```python
from build123d import *

# Parameters (mm, degrees)
F0_W          = 28.3464
F0_H          = 2.54
F0_W_2        = 2.54
F1_DEPTH      = 43.18
F2_W          = 28.3464
F2_H          = 10.16
F3_DEPTH      = 2.54
F2_W_2        = 2.54
F2_H_2        = 2.54
F4_DEPTH      = 12.7
F5_DEPTH      = 25.4
F6_W          = 33.4264
F6_H          = 22.86
F7_DEPTH      = 12.7
F9_W          = 35.56
F9_H          = 27.94
F10_DEPTH     = 25.4
F11_W         = 35.56
F11_H         = 22.86
F12_DEPTH     = 12.7
F14_W         = 36.8241928518
F14_H         = 28.1280204654
F15_DEPTH     = 25.4
F17_DEPTH     = 12.7
F19_W         = 36.3356121816
F19_H         = 38.6965835933
F20_DEPTH     = 25.4
F21_T4_DEPTH  = 37.4897748093
F21_T10_DEPTH = 37.4897748093
F22_T4_DEPTH  = 41.4622128931
F22_T9_DEPTH  = 41.4622128931
F22_T15_DEPTH = 39.215050137
F22_T21_DEPTH = 39.215050137
F22_T26_DEPTH = 13.1188216118
F23_T4_DEPTH  = 41.4622128931
F23_T9_DEPTH  = 41.4622128931
F23_T14_DEPTH = 39.215050137
F24_W         = 28.3464
F24_H         = 2.54
F25_DEPTH     = 25.4


# Not quite as in the source:
# - a fillet or chamfer that OpenCascade refuses, or shapes differently, is made with other operations: its cross-section is extruded or revolved along the edge and cut away or added


with BuildPart() as f1:
    # F0 (on Front) → F1 (new body)
    with BuildSketch(Plane.XZ):
        with Locations((16.7132, 1.27)):
            Rectangle(F0_W, F0_H)
        with Locations((1.27, 1.27)):
            Rectangle(F0_W_2, F0_H)
        with Locations((32.1564, 1.27)):
            Rectangle(F0_W_2, F0_H)
    extrude(amount=F1_DEPTH)

    # F2 (on face) → F3 (cut)
    with BuildSketch(Plane.XY.offset(2.54)):
        Polygon((30.8864, 0), (2.54, 0), (2.54, -7.62), (2.54, -27.94), (30.8864, -27.94), (30.8864, -7.62), align=None)
        with Locations((16.7132, -35.56)):
            Rectangle(F2_W, F2_H)
    extrude(amount=-F3_DEPTH, mode=Mode.SUBTRACT)

    # F2 (on face) → F4 (join)
    with BuildSketch(Plane.XY.offset(2.54)):
        with Locations((1.27, -41.91)):
            Rectangle(F2_W_2, F2_H_2)
        with Locations((32.1564, -41.91)):
            Rectangle(F2_W_2, F2_H_2)
    extrude(amount=F4_DEPTH)

    # F2 (on face) → F5 (join)
    with BuildSketch(Plane.XY.offset(2.54)):
        Polygon((2.54, -7.62), (0, -7.62), (0, -40.64), (2.54, -40.64), (2.54, -30.48), (2.54, -27.94), align=None)
        Polygon((33.4264, -7.62), (30.8864, -7.62), (30.8864, -27.94), (30.8864, -30.48), (30.8864, -40.64), (33.4264, -40.64), align=None)
        with Locations((16.7132, -41.91)):
            Rectangle(F2_W, F2_H_2)
        with Locations((1.27, -41.91)):
            Rectangle(F2_W_2, F2_H_2)
        with Locations((32.1564, -41.91)):
            Rectangle(F2_W_2, F2_H_2)
    extrude(amount=-F5_DEPTH)

    # F6 (on face) → F7 (join)
    with BuildSketch(Plane.XZ.offset(43.18)):
        with Locations((16.7132, -11.43)):
            Rectangle(F6_W, F6_H)
    extrude(amount=F7_DEPTH)

    # F9 (on 3pt) → F10 (cut)
    with BuildSketch(Plane(origin=(0, -32.9960377358, 18.3311320755), x_dir=(-1, 0, 0), z_dir=(0, 0.8741572761, -0.4856429312))):
        with Locations((-17.78, -36.665337096)):
            Rectangle(F9_W, F9_H)
    extrude(amount=-F10_DEPTH, mode=Mode.SUBTRACT)

    # F11 (on face) → F12 (join)
    with BuildSketch(Plane.YZ.offset(33.4264)):
        with Locations((-25.4, -11.43)):
            Rectangle(F11_W, F11_H)
    extrude(amount=F12_DEPTH)

    # F14 (on 3pt) → F15 (cut)
    with BuildSketch(Plane(origin=(25.5428150943, 0, 14.1904528302), x_dir=(0, -1, 0), z_dir=(-0.8741572761, 0, -0.4856429312))):
        with Locations((24.8448457569, -30.2426330745)):
            Rectangle(F14_W, F14_H)
    extrude(amount=-F15_DEPTH, mode=Mode.SUBTRACT)

    # F16 (on face) → F17 (join)
    with BuildSketch(Plane(origin=(0, 0, 0), x_dir=(0, -1, 0), z_dir=(-1, 0, 0))):
        Polygon((40.64, -22.86), (40.64, 2.54), (7.62, 2.54), (7.62, 0), (7.62, -22.86), align=None)
    extrude(amount=F17_DEPTH)

    # F19 (on 3pt) → F20 (cut)
    with BuildSketch(Plane(origin=(-1.016, 0, 0.508), x_dir=(0, -1, 0), z_dir=(-0.894427191, 0, 0.4472135955))):
        with Locations((25.5430552643, -17.0687864302)):
            Rectangle(F19_W, F19_H)
    extrude(amount=F20_DEPTH, mode=Mode.SUBTRACT)

    # F21: chamfer of 5.08 on 2 edges, made by hand


with BuildPart() as f21_tool2:
    # F21_s3 → F21_t4 (new body)
    with BuildSketch(Plane(origin=(0, -29.228474159, -52.6112534862), x_dir=(1, 0, 0), z_dir=(0, 0.4856429312, 0.8741572761))):
        with BuildLine():
            Line((-0.1436840979, -32.522427085), (5.2236840979, -37.8897952809))
            Line((5.2236840979, -37.8897952809), (5.2236840979, -37.9913952809))
            ThreePointArc((5.2236840979, -37.9913952809), (2.611842049, -37.8477111829), (0, -37.8477111829))
            Line((0, -37.8477111829), (-0.1016, -37.7461111829))
            ThreePointArc((-0.1016, -37.7461111829), (-0.1016, -35.134269134), (-0.2452840979, -32.522427085))
            Line((-0.2452840979, -32.522427085), (-0.1436840979, -32.522427085))
        make_face()
    extrude(amount=F21_T4_DEPTH)

    split(bisect_by=Plane.XY.offset(-22.86), keep=Keep.TOP)

    split(bisect_by=Plane.XZ.offset(40.64), keep=Keep.TOP)


with BuildPart() as f1_1:
    add(f1.part)

    # F21_t1: cut F21_tool2
    add(f21_tool2.part, mode=Mode.SUBTRACT)


with BuildPart() as f21_tool8:
    # F21_s9 → F21_t10 (new body)
    with BuildSketch(Plane(origin=(0, -11.0218300314, -19.8392940565), x_dir=(1, 0, 0), z_dir=(0, -0.4856429312, -0.8741572761))):
        with BuildLine():
            Line((33.5700840979, 32.522427085), (28.2027159021, 37.8897952809))
            Line((28.2027159021, 37.8897952809), (28.2027159021, 37.9913952809))
            ThreePointArc((28.2027159021, 37.9913952809), (30.814557951, 37.8477111829), (33.4264, 37.8477111829))
            Line((33.4264, 37.8477111829), (33.528, 37.7461111829))
            ThreePointArc((33.528, 37.7461111829), (33.528, 35.134269134), (33.6716840979, 32.522427085))
            Line((33.6716840979, 32.522427085), (33.5700840979, 32.522427085))
        make_face()
    extrude(amount=F21_T10_DEPTH)

    split(bisect_by=Plane.XZ.offset(43.18), keep=Keep.TOP)

    split(bisect_by=Plane.XY.offset(-22.86), keep=Keep.TOP)


with BuildPart() as f1_2:
    add(f1_1.part)

    # F21_t7: cut F21_tool8
    add(f21_tool8.part, mode=Mode.SUBTRACT)

    # F22: chamfer of 5.08 on 2 edges, made by hand


with BuildPart() as f22_tool2:
    # F22_s3 → F22_t4 (new body)
    with BuildSketch(Plane(origin=(-17.5264653053, 0, -35.0529306106), x_dir=(0, 1, 0), z_dir=(0.4472135955, 0, 0.894427191))):
        Polygon((-40.64, -3.9440774674), (-35.56, 1.1359225326), (-40.64, 1.1359225326), align=None)
    extrude(amount=F22_T4_DEPTH)

    split(bisect_by=Plane.YZ, keep=Keep.BOTTOM)


with BuildPart() as f1_3:
    add(f1_2.part)

    # F22_t1: cut F22_tool2
    add(f22_tool2.part, mode=Mode.SUBTRACT)


with BuildPart() as f22_tool7:
    # F22_s8 → F22_t9 (new body)
    with BuildSketch(Plane(origin=(-17.5264653053, 0, -35.0529306106), x_dir=(0, 1, 0), z_dir=(0.4472135955, 0, 0.894427191))):
        Polygon((-40.64, -3.9440774674), (-35.56, 1.1359225326), (-40.64, 1.1359225326), align=None)
    extrude(amount=F22_T9_DEPTH)

    split(bisect_by=Plane(origin=(-16.3330555915, -14.2776593863, 7.9320329924), x_dir=(0.6581451817, -0.7528910411, 0), z_dir=(-0.7071067812, -0.6181225378, 0.3434014099)), keep=Keep.TOP)

    split(bisect_by=Plane(origin=(0, -11.0218300314, -19.8392940565), x_dir=(1, 0, 0), z_dir=(0, -0.4856429312, -0.8741572761)), keep=Keep.TOP)


with BuildPart() as f1_4:
    add(f1_3.part)

    # F22_t6: cut F22_tool7
    add(f22_tool7.part, mode=Mode.SUBTRACT)


with BuildPart() as f22_tool13:
    # F22_s14 → F22_t15 (new body)
    with BuildSketch(Plane(origin=(26.9280968005, 0, -48.4705742409), x_dir=(0, 1, 0), z_dir=(-0.4856429312, 0, 0.8741572761))):
        Polygon((-38.1, -29.2199307745), (-43.18, -24.1399307745), (-43.18, -29.2199307745), align=None)
    extrude(amount=F22_T15_DEPTH)

    split(bisect_by=Plane(origin=(33.0462555918, -28.8876247736, 16.0486804298), x_dir=(0.6581451817, 0.7528910411, 0), z_dir=(0.7071067812, -0.6181225378, 0.3434014099)), keep=Keep.TOP)

    split(bisect_by=Plane(origin=(0, -11.0218300314, -19.8392940565), x_dir=(1, 0, 0), z_dir=(0, -0.4856429312, -0.8741572761)), keep=Keep.TOP)


with BuildPart() as f1_5:
    add(f1_4.part)

    # F22_t12: cut F22_tool13
    add(f22_tool13.part, mode=Mode.SUBTRACT)


with BuildPart() as f22_tool19:
    # F22_s20 → F22_t21 (new body)
    with BuildSketch(Plane(origin=(26.9280968005, 0, -48.4705742409), x_dir=(0, 1, 0), z_dir=(-0.4856429312, 0, 0.8741572761))):
        Polygon((-38.1, -29.2199307745), (-43.18, -24.1399307745), (-43.18, -29.2199307745), align=None)
    extrude(amount=F22_T21_DEPTH)

    split(bisect_by=Plane.YZ.offset(33.4264), keep=Keep.TOP)


with BuildPart() as f1_6:
    add(f1_5.part)

    # F22_t18: cut F22_tool19
    add(f22_tool19.part, mode=Mode.SUBTRACT)


with BuildPart() as f22_tool24:
    # F22_s25 → F22_t26 (new body)
    with BuildSketch(Plane(origin=(1.5125219245, 0, -2.7225394641), x_dir=(0, 1, 0), z_dir=(0.4856429312, 0, -0.8741572761))):
        Polygon((-38.1, 29.2199307745), (-43.18, 24.1399307745), (-43.18, 29.2199307745), align=None)
    extrude(amount=F22_T26_DEPTH)

    split(bisect_by=Plane(origin=(33.0462555918, -28.8876247736, 16.0486804298), x_dir=(0.6581451817, 0.7528910411, 0), z_dir=(0.7071067812, -0.6181225378, 0.3434014099)), keep=Keep.TOP)

    split(bisect_by=Plane(origin=(0, -11.0218300314, -19.8392940565), x_dir=(1, 0, 0), z_dir=(0, -0.4856429312, -0.8741572761)), keep=Keep.TOP)


with BuildPart() as f1_7:
    add(f1_6.part)

    # F22_t23: cut F22_tool24
    add(f22_tool24.part, mode=Mode.SUBTRACT)

    # F23: chamfer of 2.54 on 2 edges, made by hand


with BuildPart() as f23_tool2:
    # F23_s3 → F23_t4 (new body)
    with BuildSketch(Plane(origin=(3.9372326527, 0, 7.8744653053), x_dir=(0, 1, 0), z_dir=(-0.4472135955, 0, -0.894427191))):
        Polygon((-10.16, -1.1359225326), (-7.62, 1.4040774674), (-7.62, -1.1359225326), align=None)
    extrude(amount=F23_T4_DEPTH)

    split(bisect_by=Plane.XY, keep=Keep.BOTTOM)


with BuildPart() as f1_8:
    add(f1_7.part)

    # F23_t1: cut F23_tool2
    add(f23_tool2.part, mode=Mode.SUBTRACT)


with BuildPart() as f23_tool7:
    # F23_s8 → F23_t9 (new body)
    with BuildSketch(Plane(origin=(3.9372326527, 0, 7.8744653053), x_dir=(0, 1, 0), z_dir=(-0.4472135955, 0, -0.894427191))):
        Polygon((-10.16, -1.1359225326), (-7.62, 1.4040774674), (-7.62, -1.1359225326), align=None)
    extrude(amount=F23_T9_DEPTH)

    split(bisect_by=Plane.YZ, keep=Keep.BOTTOM)


with BuildPart() as f1_9:
    add(f1_8.part)

    # F23_t6: cut F23_tool7
    add(f23_tool7.part, mode=Mode.SUBTRACT)


with BuildPart() as f23_tool12:
    # F23_s13 → F23_t14 (new body)
    with BuildSketch(Plane(origin=(23.7558408531, 0, -42.7605135355), x_dir=(0, 1, 0), z_dir=(-0.4856429312, 0, 0.8741572761))):
        Polygon((-7.62, -26.6799307745), (-10.16, -29.2199307745), (-7.62, -29.2199307745), align=None)
    extrude(amount=F23_T14_DEPTH)

    split(bisect_by=Plane.XY, keep=Keep.BOTTOM)


with BuildPart() as f1_10:
    add(f1_9.part)

    # F23_t11: cut F23_tool12
    add(f23_tool12.part, mode=Mode.SUBTRACT)

    # F24 (on face) → F25 (join)
    with BuildSketch(Plane.XY.offset(2.54)):
        with Locations((16.7132, -29.21)):
            Rectangle(F24_W, F24_H)
    extrude(amount=-F25_DEPTH)


solid = f1_10.part
```
Verification items for the finished model (mm, model axes). A direction names the side the tool comes from. Coordinates: 2 decimals unless noted, no trailing zeros. Loops run counter-clockwise (first coordinate to the right, second up) from the corner with the lowest first, then second, coordinate; pieces in that order, holes last. Notation, with made-up numbers: (13, 16.25) - (68, 16.25) arc R16 cw to (68, 27.25) - close; hole circle Ø4 at (5.5, -13.5). An arc over 180 degrees is marked (long way). Return JSON: item names as keys, results as strings.
1. Go/stop test with flat-tipped pins: pin 1 (1.3 mm diameter, centred on y = -42.5, z = 10, fed in from -X); pin 2 (4 mm diameter, centred on x = 6, y = -7.5, fed in from +Z); pin 3 (3.5 mm diameter, centred on x = -6.5, z = -12, fed in from +Y); pin 4 (3 mm diameter, centred on y = -34, z = -7, fed in from -X). Record where each tip stops, or that it passes through.
Established:
{"pin 1": "stops at x = 0", "pin 2": "passes through", "pin 3": "stops at y = -7.72", "pin 4": "stops at x = -5.52"}
2. Section check C-C, the plane z = -20. Record the boundary of the cut face in (x, y), then the cut area to 3 significant figures.
Established:
{"outline": "(-11.27, -35.56) - (-5.59, -40.64) - (0, -40.64) - (0, -48.48) - (5.08, -54.29) - (28.35, -54.29) - (33.43, -48.48) - (33.43, -43.18) - (38.73, -43.18) - (44.54, -38.1) - (44.54, -10.16) - (41.63, -7.62) - (30.89, -7.62) - (30.89, -27.94) - (2.54, -27.94) - (2.54, -7.62) - (-8.43, -7.62) - (-11.27, -10.16) - close; hole (2.54, -40.64) - (30.89, -40.64) - (30.89, -30.48) - (2.54, -30.48) - close", "area": "1,400 mm2"}
3. Tool access check on faces 5 (the flat face through (33.426, -26, 1)), 6 (the flat face through (0, -43, -13)), 7 (the flat face through (16.876, -49.866, -12.035)), 8 (the flat face through (33.426, -41, -1)). Record the directions out of +Z, -Z, +X, -X, +Y, -Y that give a thin tool (end or side, any length) a straight path to the whole face; none if there is none.
Established:
{"face 5": "+Z, +X, +Y, -Y", "face 6": "+Z, -X, -Y", "face 7": "+X, -X, -Y", "face 8": "+Z, +X, -Y"}
4. Mould release check, pull along Z, two halves, no side actions. Record for faces 1 (the flat face through (17, -30.48, -10)), 2 (the flat face through (32, -5, 0)), 3 (the flat face through (-4.64, -37.57, -11.24)), 4 (the flat face through (16.947, -44.695, -1.132)): +Z half, -Z half, draft (parallel to the pull), parting line (faces both ways), or undercut.
Established:
{"face 1": "draft", "face 2": "undercut", "face 3": "+Z half", "face 4": "undercut"}
5. Section check A-A, the plane z = 8. Record the boundary of the cut face in (x, y), then the cut area to 3 significant figures.
Established:
{"outline": "(0, -43.18) - (2.54, -43.18) - (2.54, -40.64) - (0, -40.64) - close; (30.89, -43.18) - (33.43, -43.18) - (33.43, -40.64) - (30.89, -40.64) - close", "area": "12.9 mm2"}
6. Section check D-D, the plane x = 35.5. Record the boundary of the cut face in (y, z).
Established:
{"outline": "(-43.18, -22.86) - (-7.62, -22.86) - (-7.62, -8.96) - (-10.16, -3.73) - (-38.1, -3.73) - (-43.18, -14.19) - close"}
7. Thickness scan on L1, parallel to Y at x = 18.5, z = 2.5; L2, parallel to X at y = -15, z = -1.5; L3, parallel to Y at x = -5, z = -21. Record the ranges inside material, lowest first.
Established:
{"L1": "y = -43.18 to -40.64, -30.48 to -27.94", "L2": "x = -2.02 to 2.54, 30.89 to 34.26", "L3": "y = -40.64 to -7.62"}
